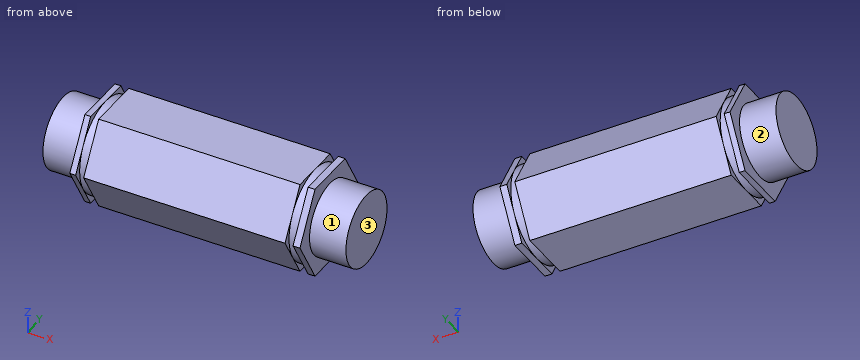
Autodesk Inventor part; units mm, degrees
ref_plane "Work Plane1" through (34.549, -3.6662, -6.35) normal (1, 0, 0) x (0, 0, -1)
ref_plane "Work Plane2" through (6.9, -3.6662, 6.35) normal (-1, 0, 0) x (0, 0, 1)
ref_plane "YZ Plane" through (0, 0, 0) normal (1, 0, 0) x (0, 1, 0)
sketch "Sketch1" plane through (0, 0, 0) normal (0, 0, 1) x (1, 0, 0)
  line L0 (0, 0) -> (0, 5)
  line L1 (0, 5) -> (5, 5)
  line L2 (5, 5) -> (5, 8.4186)
  line L3 (5, 8.4186) -> (36.6, 8.4186)
  line L4 (36.6, 8.4186) -> (36.6, 5)
  line L5 (36.6, 5) -> (41.6, 5)
  line L6 (41.6, 5) -> (41.6, 0)
  line L7 (41.6, 0) -> (0, 0)
  dimension "d0" = 31.6
  dimension "d1" = 5
  dimension "d2" = 5
  dimension "d3" = 5
revolve "Revolution1" add sketch "Sketch1" angle 360 about axis through (41.6, 0, 0) along (-1, 0, 0)
sketch "Sketch2" plane through (36.6, 0, 0) normal (1, 0, 0) x (0, 0, -1)
  circle A0 centre (0, 0) radius 5
  line L0 (0, 7.3323) -> (6.35, 3.6662)
  line L1 (6.35, 3.6662) -> (6.35, -3.6662)
  line L2 (6.35, -3.6662) -> (0, -7.3323)
  line L3 (0, -7.3323) -> (-6.35, -3.6662)
  line L4 (-6.35, -3.6662) -> (-6.35, 3.6662)
  line L5 (-6.35, 3.6662) -> (0, 7.3323)
  circle A1 centre (0, 0) radius 5
  circle A2 centre (0, 0) radius 8.4186
  dimension "d5" = 12.7
extrude "Extrusion1" cut sketch "Sketch2" against normal up to surface (31.6 mm away) contours A2
ref_plane "Work Plane1" through (34.549, -3.6662, -6.35) normal (1, 0, 0) x (0, 0, -1)
sketch "Sketch3" plane through (34.549, -3.6662, -6.35) normal (1, 0, 0) x (0, 0, -1)
  circle A0 centre (-6.35, 3.6662) radius 5
  circle A1 centre (-6.35, 3.6662) radius 6.35
  line L0 (0, 7.3323) -> (-6.35, 10.9985)
  circle A2 centre (-6.35, 3.6662) radius 5.85
  line L1 (-6.35, -3.6662) -> (0, 0)
  line L2 (0, 0) -> (0, 7.3323)
  line L3 (0, 7.3323) -> (-6.35, 10.9985)
  line L4 (-6.35, 10.9985) -> (-12.7, 7.3323)
  line L5 (-12.7, 7.3323) -> (-12.7, 0)
  line L6 (-12.7, 0) -> (-6.35, -3.6662)
  circle A3 centre (-6.35, 3.6662) radius 5
  dimension "d9" = 0.5
extrude "Extrusion2" cut sketch "Sketch3" along normal blind 1.1 contours L2 L1 A1 | A1 L0 L2 | A1 L4 L0 | L1 L6 A1 | A1 L5 L4 | L6 L5 A1
ref_plane "Work Plane2" through (6.9, -3.6662, 6.35) normal (-1, 0, 0) x (0, 0, 1)
sketch "Sketch4" plane through (6.9, -3.6662, 6.35) normal (-1, 0, 0) x (0, 0, 1)
  line L0 (-12.7, 0) -> (-6.35, -3.6662)
  line L1 (-6.35, -3.6662) -> (0, 0)
  line L2 (0, 0) -> (0, 7.3323)
  line L3 (0, 7.3323) -> (-6.35, 10.9985)
  line L4 (-6.35, 10.9985) -> (-12.7, 7.3323)
  line L5 (-12.7, 7.3323) -> (-12.7, 0)
  circle A0 centre (-6.35, 3.6662) radius 5
  circle A1 centre (-6.35, 3.6662) radius 5
  circle A2 centre (-6.35, 3.6662) radius 6.35
extrude "Extrusion3" cut sketch "Sketch4" along normal blind 1.1 contours L5 A2 L0 | A2 L1 L0 | L5 L4 A2 | A2 L2 L1 | L4 L3 A2 | A2 L3 L2
properties part number "Hex Shaft 1" material "Steel, Mild"
Source: CAD feature listing. Evaluate the final solid. Frame: model axes, mm. Face numbers are marked on the shaded views. A direction names the side the tool comes from. Coordinates: 2 decimals unless noted, no trailing zeros. Write each loop counter-clockwise with the first axis right and the second up, starting at its lowest first coordinate (ties: lowest second). Pieces come first, ordered by that corner, then holes. Notation, with made-up numbers: (46, 8.5) - (57, 8.5) arc R15 ccw to (57, 24.5) - close; hole circle Ø3 at (30, 23.5). An arc over 180 degrees is marked (long way). Answer as a JSON object with one key per item and string values.
Q1. Section query B-B, the plane y = -1.75. Output: boundary loops of the cut face in (x, z).
Ans:
{"outline": "(0, -4.68) - (5, -4.68) - (5, -6.35) - (5.8, -6.35) - (5.8, -6.1) - (6.9, -6.1) - (6.9, -6.35) - (34.55, -6.35) - (34.55, -6.1) - (35.65, -6.1) - (35.65, -6.35) - (36.6, -6.35) - (36.6, -4.68) - (41.6, -4.68) - (41.6, 4.68) - (36.6, 4.68) - (36.6, 6.35) - (35.65, 6.35) - (35.65, 6.1) - (34.55, 6.1) - (34.55, 6.35) - (6.9, 6.35) - (6.9, 6.1) - (5.8, 6.1) - (5.8, 6.35) - (5, 6.35) - (5, 4.68) - (0, 4.68) - close"}
Q2. Section query C-C, the plane x = 35. Output: boundary loops of the cut face in (y, z).
Ans:
{"outline": "circle Ø12.7 at (0, 0)"}
Q3. Material intervals for line 1 (X direction, y = -4.5, z = -2.25); line 2 (Y direction, x = 8.5, z = -4.25); line 3 (Y direction, x = 19.5, z = -3.5), sorted ascending. Write a range as [from, to].
Ans:
{"line 1": "x = [5, 36.6]", "line 2": "y = [-4.88, 4.88]", "line 3": "y = [-5.31, 5.31]"}
Q4. Section query A-A, the plane z = 0.5. Output: boundary loops of the cut face in (x, y), plus the area to 3 significant figures.
Ans:
{"outline": "(0, -4.97) - (5, -4.97) - (5, -7.04) - (5.8, -7.04) - (5.8, -6.33) - (6.9, -6.33) - (6.9, -7.04) - (34.55, -7.04) - (34.55, -6.33) - (35.65, -6.33) - (35.65, -7.04) - (36.6, -7.04) - (36.6, -4.97) - (41.6, -4.97) - (41.6, 4.97) - (36.6, 4.97) - (36.6, 7.04) - (35.65, 7.04) - (35.65, 6.33) - (34.55, 6.33) - (34.55, 7.04) - (6.9, 7.04) - (6.9, 6.33) - (5.8, 6.33) - (5.8, 7.04) - (5, 7.04) - (5, 4.97) - (0, 4.97) - close", "area": "542 mm2"}
Q5. Section query D-D, the plane x = 27. Output: boundary loops of the cut face in (y, z), plus the area to 3 significant figures.
Ans:
{"outline": "(-7.33, 0) - (-3.67, -6.35) - (3.67, -6.35) - (7.33, 0) - (3.67, 6.35) - (-3.67, 6.35) - close", "area": "140 mm2"}
Q6. Set-up query: the marked faces 1, 2 and 3. Return all of +Z, -Z, +X, -X, +Y, -Y with unobstructed straight access to the full face (end or side cutting, diameter ignored); none if empty.
Ans:
{"face 1": "+X", "face 2": "-X", "face 3": "+Z, -Z, +X, +Y, -Y"}
Q7. First-contact query: pin 1 Ø0.5 at (y, z) = (-6.5, -1) entering from -X; pin 2 Ø1 at (y, z) = (3.5, -4.5) entering from +X. Flat tips, straight axial feed; report the tip coordinate or a pass-through.
Ans:
{"pin 1": "stops at x = 5", "pin 2": "stops at x = 36.6"}
